Can you work these out from the model? Positions are in its coordinate system, mm. A direction names the side the tool comes from. Coordinates: 2 decimals unless noted, no trailing zeros. Order: outer loops, then holes, each group sorted by start corner. A loop starts at its lowest first (then second) coordinate and runs counter-clockwise, first axis right, second up. Notation, with made-up numbers: (8, 27) -> (17, 27) arc R26 ccw to (17, 42) -> close; hole circle Ø2 at (50.5, 16). An arc over 180 degrees is marked (long way). Answer in a Markdown table with one row per item.
```python
from build123d import *

# Parameters (mm, degrees)
BOSS_EXTRUDE1_DEPTH = 9.5
SKETCH5_W           = 107.5
SKETCH5_H           = 25
BOSS_EXTRUDE4_DEPTH = 15
BOSS_EXTRUDE5_DEPTH = 13
SKETCH7_W           = 6.5
SKETCH7_H           = 11.5
CUT_EXTRUDE1_DEPTH  = 169.774998148
FILLET1_R           = 2.5


with BuildPart() as part:
    # Sketch1 → Boss-Extrude1 (new, symmetric)
    with BuildSketch(Plane.XY):
        Polygon((0, 0), (-138, 0), (-138, 96), (0, 96), (0, 86), (-22.96030313, 60.5), (-30.5, 60.5), (-30.5, 35.5), (-22.96030313, 35.5), (0, 10), align=None)
        with BuildLine():
            Line((-107.5, 84), (-57.5, 84))
            ThreePointArc((-57.5, 84), (-52, 78.5), (-57.5, 73))
            Line((-57.5, 73), (-107.5, 73))
            ThreePointArc((-107.5, 73), (-113, 78.5), (-107.5, 84))
        make_face(mode=Mode.SUBTRACT)
        with BuildLine():
            Line((-107.5, 23), (-57.5, 23))
            ThreePointArc((-57.5, 23), (-52, 17.5), (-57.5, 12))
            Line((-57.5, 12), (-107.5, 12))
            ThreePointArc((-107.5, 12), (-113, 17.5), (-107.5, 23))
        make_face(mode=Mode.SUBTRACT)
    extrude(amount=BOSS_EXTRUDE1_DEPTH, both=True)

    # Sketch5 → Boss-Extrude4 (add, symmetric)
    with BuildSketch(Plane.XY):
        with Locations((-84.25, 48)):
            Rectangle(SKETCH5_W, SKETCH5_H)
    extrude(amount=BOSS_EXTRUDE4_DEPTH, both=True)

    # Sketch6 → Boss-Extrude5 (add, symmetric)
    with BuildSketch(Plane.XY):
        Polygon((-6.30282831, 79), (-35, 79), (-35, 96), (0, 96), (0, 86), align=None)
        Polygon((-6.30282831, 17), (-35, 17), (-35, 0), (0, 0), (0, 10), align=None)
    extrude(amount=BOSS_EXTRUDE5_DEPTH, both=True)

    # Sketch7 → Cut-Extrude1 (cut, through all)
    with BuildSketch(Plane(origin=(0, 96, 0), x_dir=(1, 0, 0), z_dir=(0, 1, 0))):
        with Locations((-134.75, -9.25)):
            Rectangle(SKETCH7_W, SKETCH7_H)
    extrude(amount=-CUT_EXTRUDE1_DEPTH, mode=Mode.SUBTRACT)

    # Fillet1
    fillet1_edges = [part.edges().sort_by_distance(p)[0] for p in [
        (-113, 78.5, -9.5),
        (-82.5, 73, -9.5),
        (-52, 78.5, -9.5),
        (-82.5, 84, -9.5),
        (-113, 78.5, 9.5),
        (-82.5, 73, 9.5),
        (-52, 78.5, 9.5),
        (-82.5, 84, 9.5),
        (-113, 17.5, -9.5),
        (-82.5, 12, -9.5),
        (-52, 17.5, -9.5),
        (-82.5, 23, -9.5),
        (-113, 17.5, 9.5),
        (-82.5, 12, 9.5),
        (-52, 17.5, 9.5),
        (-82.5, 23, 9.5),
    ]]
    fillet(fillet1_edges, radius=FILLET1_R)


solid = part.part
```
(1) Suppose I cut it at A-A (x = -105.5). Please give me the cut outline in (y, z).
Response values:
| item | result |
|---|---|
| outline | (0, -9.5) -> (9.5, -9.5) arc R2.5 ccw to (12, -7) -> (12, 7) arc R2.5 ccw to (9.5, 9.5) -> (0, 9.5) -> close; (23, -7) arc R2.5 ccw to (25.5, -9.5) -> (35.5, -9.5) -> (35.5, -15) -> (60.5, -15) -> (60.5, -9.5) -> (70.5, -9.5) arc R2.5 ccw to (73, -7) -> (73, 7) arc R2.5 ccw to (70.5, 9.5) -> (60.5, 9.5) -> (60.5, 15) -> (35.5, 15) -> (35.5, 9.5) -> (25.5, 9.5) arc R2.5 ccw to (23, 7) -> close; (84, -7) arc R2.5 ccw to (86.5, -9.5) -> (96, -9.5) -> (96, 9.5) -> (86.5, 9.5) arc R2.5 ccw to (84, 7) -> close |
(2) I need wall thicknesses on line 1 (Y direction, x = -79, z = -6.75); line 2 (Y direction, x = -15, z = 10.75); line 3 (Y direction, x = -110.5, z = 9). Which ranges of each line are inside material? Lowest first, please. Write a range as [from, to].
Response values:
| item | result |
|---|---|
| line 1 | [0, 12], [23, 73], [84, 96] |
| line 2 | [0, 17], [79, 96] |
| line 3 | [0, 11.73], [23.27, 72.73], [84.27, 96] |
(3) Suppose I cut it at C-C (z = -5). Please give me the cut outline in (x, y), and give its area (3 significant figures).
Response values:
| item | result |
|---|---|
| outline | (-138, 0) -> (0, 0) -> (0, 10) -> (-22.96, 35.5) -> (-30.5, 35.5) -> (-30.5, 60.5) -> (-22.96, 60.5) -> (0, 86) -> (0, 96) -> (-138, 96) -> close; hole (-107.5, 12) -> (-57.5, 12) arc R5.5 ccw to (-57.5, 23) -> (-107.5, 23) arc R5.5 ccw to start; hole (-107.5, 73) -> (-57.5, 73) arc R5.5 ccw to (-57.5, 84) -> (-107.5, 84) arc R5.5 ccw to start |
| area | 10,600 mm2 |
(4) Will these pins go through, and if not, where does the flat tip stop? pin 1 Ø18.5 at (x, y) = (-17.5, 89) entering from -Z; pin 2 Ø1 at (y, z) = (5.5, -10.5) entering from -X; pin 3 Ø6 at (x, y) = (-63.5, 70) entering from +Z.
Response values:
| item | result |
|---|---|
| pin 1 | z = -13 |
| pin 2 | x = -35 |
| pin 3 | z = 9.5 |
(5) Suppose I cut it at D-D (x = -127). Please give me the cut outline in (y, z), and give its area (3 significant figures).
Response values:
| item | result |
|---|---|
| outline | (0, -9.5) -> (35.5, -9.5) -> (35.5, -15) -> (60.5, -15) -> (60.5, -9.5) -> (96, -9.5) -> (96, 9.5) -> (60.5, 9.5) -> (60.5, 15) -> (35.5, 15) -> (35.5, 9.5) -> (0, 9.5) -> close |
| area | 2,100 mm2 |
(6) We'd pull the mould along Y, two halves only. Please class faces 1 (the flat face through (-68, 0, 0)), 2 (the flat face through (-85, 48, -15)), 3 (the flat face through (-83, 84, 0)): +Y half, -Y half, draft (parallel to the pull), parting line (faces both ways), or undercut.
Response values:
| item | result |
|---|---|
| face 1 | -Y half |
| face 2 | draft |
| face 3 | undercut |
(7) Suppose I cut it at B-B (z = -11.5). Please give me the cut outline in (x, y), and give its area (3 significant figures).
Response values:
| item | result |
|---|---|
| outline | (-138, 35.5) -> (-30.5, 35.5) -> (-30.5, 60.5) -> (-138, 60.5) -> close; (-35, 0) -> (0, 0) -> (0, 10) -> (-6.3, 17) -> (-35, 17) -> close; (-35, 79) -> (-6.3, 79) -> (0, 86) -> (0, 96) -> (-35, 96) -> close |
| area | 3,830 mm2 |
(8) On a 3-axis mill with a long thin cutter (end or side, diameter ignored), from which of +Z, -Z, +X, -X, +Y, -Y can I reach the whole of each face in a straight line? I mean faces 4 (the flat face through (-131.5, 49, 8)), 5 (the cylindrical face through (-113, 17.4, 0.1)), 6 (the flat face through (-27, 35.5, 0)). Say none if no direction works.
Response values:
| item | result |
|---|---|
| face 4 | +Z, -X, +Y, -Y |
| face 5 | +Z, -Z |
| face 6 | +Z, -Z, +X |
